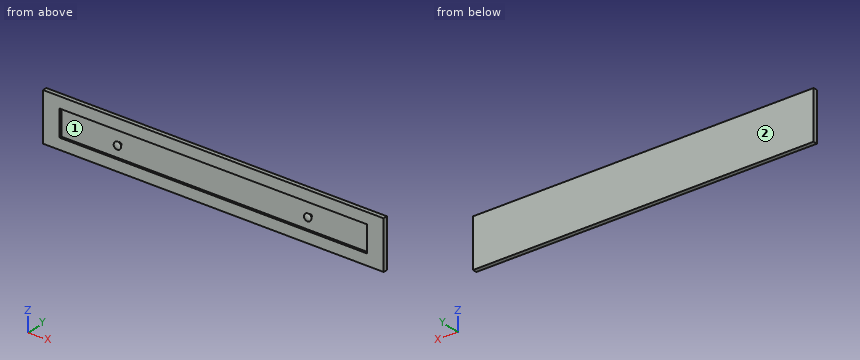
```python
from build123d import *

# Parameters (mm, degrees)
CLONE2D007_W    = 1540
CLONE2D007_H    = 219
PAD013_DEPTH    = 19
SKETCH034_W     = 1390
SKETCH034_H     = 119
POCKET013_DEPTH = 10


with BuildPart() as part:
    # Clone2D007 → Pad013 (new body)
    with BuildSketch(Plane.XZ):
        with Locations((770, 109.5)):
            Rectangle(CLONE2D007_W, CLONE2D007_H)
    extrude(amount=PAD013_DEPTH)

    # Sketch034 (on Face6 of Pad013) → Pocket013 (cut)
    with BuildSketch(Plane.XZ.offset(19)):
        with Locations((770, 109.5)):
            Rectangle(SKETCH034_W, SKETCH034_H)
    extrude(amount=-POCKET013_DEPTH, mode=Mode.SUBTRACT)

    # Clone2D009 → Revolution004 (revolve)
    with BuildSketch(Plane(origin=(340, -9, 109.5), x_dir=(1, 0, 0), z_dir=(0, 0, 1))):
        with BuildLine():
            Line((0, 0), (0, -20))
            add(Edge.make_bspline(
                [(0, -20), (-18, -20), (-18, -9.133286), (-4.506424, -9.133286), (-7.5, 0)],
                knots=[0, 0, 0, 0, 0.5, 1, 1, 1, 1], degree=3, weights=[7, 6.116989, 5.810816, 6.060123, 5.999522]))
            Line((-7.5, 0), (0, 0))
        make_face()
    revolve(axis=Axis((340, -9, 109.5), (0, 1, 0)))

    # Clone2D008 → Revolution010 (revolve)
    with BuildSketch(Plane(origin=(1200, -9, 109.5), x_dir=(1, 0, 0), z_dir=(0, 0, 1))):
        with BuildLine():
            Line((0, 0), (0, -20))
            add(Edge.make_bspline(
                [(0, -20), (-18, -20), (-18, -9.133286), (-4.506424, -9.133286), (-7.5, 0)],
                knots=[0, 0, 0, 0, 0.5, 1, 1, 1, 1], degree=3, weights=[7, 6.116989, 5.810816, 6.060123, 5.999522]))
            Line((-7.5, 0), (0, 0))
        make_face()
    revolve(axis=Axis((1200, -9, 109.5), (0, 1, 0)))


with BuildPart() as part_1:
    # Body015 placement: moved
    add(part.part.moved(Location((10, -1, 675))))


solid = part_1.part
```
Source: CAD feature listing. Evaluate the final solid. Frame: model axes, mm. Face numbers are marked on the shaded views. Round coordinates to 2 decimals unless told otherwise and drop trailing zeros. Write each loop counter-clockwise with the first axis right and the second up, starting at its lowest first coordinate (ties: lowest second). Pieces come first, ordered by that corner, then holes. Notation, with made-up numbers: M 32.5,-11.5 L 38.5,-11.5 A23 ccw 38.5,9.5 Z; hole C -0.75,-23.5 d7. An arc over 180 degrees is marked long. Use CSV: the item, a comma, the result in double quotes. Start each with the question number.
Q1. First-contact query: P1, Ø8, axis at x = 616, y = -27, coming from the -Z side; P2, Ø10, axis at x = 311.5, z = 779, coming from the -Y side. Flat tips, straight axial feed; report the tip coordinate or a pass-through.
Q2. Pull-direction query (Z, two-part tool) for the marked faces 1 and 2; classes: +Z half, -Z half, draft (parallel to the pull), parting line (faces both ways), or undercut.
Q3. Line query: line 1 (X direction, y = -11.75, z = 820.5); line 2 (Z direction, x = 1353.5, y = -18); line 3 (Y direction, x = 140, z = 814). Output: solid intervals per line, ascending. Write a range as from..to.
Q4. Cut plane B-B on z = 818. Output: boundary loops of the cut face in (x, y), plus the area to 3 significant figures.
Q5. Cut plane C-C on z = 711.5. Output: boundary loops of the cut face in (x, y).
Q6. Cut plane A-A on x = 156. Output: boundary loops of the cut face in (y, z).
Results found:
1,P1,"through"
1,P2,"y = -10"
2,face 1,"undercut"
2,face 2,"draft"
3,line 1,"10..85, 1475..1550"
3,line 2,"675..725, 844..894"
3,line 3,"-10..-1"
4,outline,"M 10,-20 L 85,-20 L 85,-10 L 1475,-10 L 1475,-20 L 1550,-20 L 1550,-1 L 10,-1 Z"
4,area,"15,400 mm^2"
5,outline,"M 10,-20 L 1550,-20 L 1550,-1 L 10,-1 Z"
6,outline,"M -20,675 L -1,675 L -1,894 L -20,894 L -20,844 L -10,844 L -10,725 L -20,725 Z"
